Can you work these out from the model? Positions are in its coordinate system, mm. Face numbers are marked on the shaded views. Give positions to 0.01 mm unless a question says otherwise; leave off trailing zeros. Write each loop counter-clockwise with the first axis right and the second up, starting at its lowest first coordinate (ties: lowest second). Pieces come first, ordered by that corner, then holes.
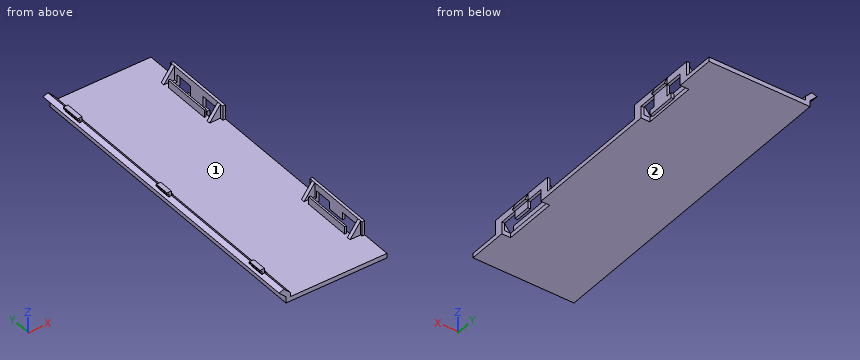
Autodesk Fusion 360 part; units mm, degrees
sketch "Sketch1" plane through (0, 0, 0) normal (0, 0, 1) x (1, 0, 0)
  line L0 (27, 90) -> (-27, 90)
  line L1 (-27, 90) -> (-27, -90)
  line L2 (-27, -90) -> (27, -90)
  line L3 (27, -90) -> (27, 90)
  dimension "d1" = 54
  dimension "d2" = 180
extrude "Extrude1" add sketch "Sketch1" along normal blind 2.5
sketch "Sketch2" plane through (0, 90, 0) normal (0, 1, 0) x (-1, 0, 0)
  line L0 (-27, 0) -> (27, 0)
  line L1 (27, 0) -> (27, 2.5)
  line L2 (27, 2.5) -> (-27, 2.5)
  line L3 (-27, 2.5) -> (-27, 0)
  line L4 (27, 0) -> (29.5, 0)
  line L5 (29.5, 0) -> (29.5, 2.5)
  line L6 (27, 2.5) -> (27, 4.8)
  line L7 (29.5, 0) -> (29.5, 3.5)
  line L8 (29.5, 3.5) -> (33.3891, 7.3891)
  line L9 (27, 4.8) -> (30.5355, 8.3355)
  line L10 (27, 4.8) -> (32.5, 4.8) construction
  line L11 (30.5355, 8.3355) -> (33.3891, 7.3891)
  dimension "d5" = 2.5
  dimension "d6" = 2.5
  dimension "d7" = 2.3
  dimension "d8" = 135
  dimension "d9" = 5.5
  dimension "d10" = 45
  dimension "d11" = 5
extrude "Extrude2" add sketch "Sketch2" against normal blind 180 contours L1 L4 L5 L6 L7 L8 L9 L11
sketch "Sketch3" plane through (0, 90, 0) normal (0, 1, 0) x (-1, 0, 0)
  line L0 (-27, 0) -> (29.5, 0)
  line L1 (29.5, 0) -> (29.5, 3.5)
  line L2 (29.5, 3.5) -> (33.3891, 7.3891)
  line L3 (33.3891, 7.3891) -> (30.5355, 8.3355)
  line L4 (30.5355, 8.3355) -> (27, 4.8)
  line L5 (27, 4.8) -> (27, 2.5)
  line L6 (27, 2.5) -> (-27, 2.5)
  line L7 (-27, 2.5) -> (-27, 0)
  line L8 (31.8891, 8.3429) -> (31.8891, 7.8866)
  line L9 (31.8891, 8.3429) -> (31.8891, 9.8429)
  line L10 (31.8891, 9.8429) -> (33.0391, 9.8429)
  line L11 (33.1891, 9.9929) -> (33.1891, 10.6929)
  line L12 (33.0391, 10.8429) -> (30.5355, 10.8429)
  line L13 (30.5355, 10.8429) -> (30.5355, 8.3355)
  arc A0 (33.1891, 10.6929) -> (33.0391, 10.8429) centre (33.0391, 10.6929) ccw
  arc A1 (33.0391, 9.8429) -> (33.1891, 9.9929) centre (33.0391, 9.9929) ccw
  line L14 (30.5355, 10.8429) -> (27, 4.8)
  point P0 (33.1891, 9.8429)
  point P1 (33.1891, 10.8429)
  dimension "d15" = 1.5
  dimension "d16" = 1.3
  dimension "d17" = 1
  dimension "d19" = 0.15
  dimension "d24" = 1.5
extrude "Extrude3" add sketch "Sketch3" along normal blind -26 and the other way blind 15.2 contours L3 L8 L9 L10 L11 L12 L13 A0 A1
extrude "Extrude4" add sketch "Sketch3" along normal blind -20 and the other way blind 22 contours L4 L13 L14
extrude "Extrude5" add sketch "Sketch3" along normal blind -94 and the other way blind 86 contours L3 L8 L9 L10 L11 L12 L13 A0 A1
extrude "Extrude6" add sketch "Sketch3" along normal blind -157 and the other way blind 165 contours L3 L8 L9 L10 L11 L12 L13 A0 A1
extrude "Extrude7" add sketch "Sketch3" along normal blind -162 and the other way blind 160 contours L4 L13 L14
extrude "Extrude8" add sketch "Sketch3" along normal blind -89 and the other way blind 91 contours L4 L13 L14
sketch "Sketch4" plane through (27, 0, 0) normal (1, 0, 0) x (0, 0, -1)
  line L0 (0, -90) -> (0, 90)
  line L1 (0, 90) -> (-2.5, 90)
  line L2 (-2.5, 90) -> (-2.5, -90)
  line L3 (-2.5, -90) -> (0, -90)
  line L4 (-2.5, -90) -> (-2.5, -73)
  line L5 (-2.5, -73) -> (-10.5, -73)
  line L6 (-10.5, -73) -> (-10.5, -33.2)
  line L7 (-2.5, -73) -> (-2.5, -68)
  line L8 (-2.5, -68) -> (-6.7, -68)
  line L9 (-10.5, -33.2) -> (-2.5, -33.2)
  line L10 (-6.7, -68) -> (-6.7, -58)
  line L11 (-6.7, -58) -> (-0.2, -58)
  line L12 (-0.2, -58) -> (-0.2, -61.1)
  line L13 (-0.2, -61.1) -> (2.7, -61.1)
  line L14 (2.7, -61.1) -> (2.7, -45.1)
  line L15 (-0.2, -48.2) -> (-0.2, -45.1)
  line L16 (-0.2, -45.1) -> (2.7, -45.1)
  line L17 (-6.7, -48.2) -> (-0.2, -48.2)
  line L18 (-6.7, -38.2) -> (-6.7, -48.2)
  line L19 (-2.5, -33.2) -> (-2.5, -38.2)
  line L20 (-2.5, -38.2) -> (-6.7, -38.2)
  line L21 (2.7, -61.1) -> (2.7, -69)
  line L22 (-2.5, -68) -> (2.7, -68)
  line L23 (-2.5, -38.2) -> (3, -38.2)
  line L24 (2.7, -45.1) -> (2.7, -38.2)
  line L25 (-1.75, 0) -> (-22.5, 0)
  line L26 (-0.2, 48.2) -> (-0.2, 45.1)
  line L27 (-0.2, 61.1) -> (2.7, 61.1)
  line L28 (-10.5, 73) -> (-10.5, 33.2)
  line L29 (-0.2, 58) -> (-0.2, 61.1)
  line L30 (-2.5, 38.2) -> (3, 38.2)
  line L31 (2.7, 61.1) -> (2.7, 69)
  line L32 (-6.7, 68) -> (-6.7, 58)
  line L33 (2.7, 61.1) -> (2.7, 45.1)
  line L34 (-6.7, 38.2) -> (-6.7, 48.2)
  line L35 (2.7, 45.1) -> (2.7, 38.2)
  line L36 (-10.5, 33.2) -> (-2.5, 33.2)
  line L37 (-2.5, 68) -> (-6.7, 68)
  line L38 (-2.5, 73) -> (-2.5, 68)
  line L39 (-6.7, 48.2) -> (-0.2, 48.2)
  line L40 (-0.2, 45.1) -> (2.7, 45.1)
  line L41 (-2.5, 68) -> (2.7, 68)
  line L42 (-2.5, 38.2) -> (-6.7, 38.2)
  line L43 (-2.5, 33.2) -> (-2.5, 38.2)
  line L44 (-2.5, 73) -> (-10.5, 73)
  line L45 (-6.7, 58) -> (-0.2, 58)
  dimension "d45" = 17
  dimension "d46" = 8
  dimension "d47" = 39.8
  dimension "d48" = 4.2
  dimension "d50" = 6.5
  dimension "d51" = 3.1
  dimension "d52" = 2.9
extrude "Extrude9" cut sketch "Sketch4" against normal blind 4.9 contours L0 L2 L11 L12 L13 L22 | L0 L13 L21 L22 | L0 L2 L11 L12 L13 L15 L16 L17 | L0 L13 L14 L16 | L2 L8 L10 L11 | L0 L2 L15 L16 L17 L23 | L0 L16 L23 L24 | L2 L17 L18 L20 | L0 L2 L26 L30 L39 L40 | L0 L30 L35 L40 | L0 L2 L26 L27 L29 L39 L40 L45 | L0 L27 L33 L40 | L2 L34 L39 L42 | L0 L2 L27 L29 L41 L45 | L0 L27 L31 L41 | L2 L32 L37 L45
extrude "Extrude10" add sketch "Sketch4" against normal blind 1.5 contours L0 L2 L11 L12 L13 L15 L16 L17 | L0 L13 L14 L16 | L2 L5 L6 L7 L8 L9 L10 L11 L17 L18 L19 L20
sketch "Sketch5" plane through (0, -73, 0) normal (0, -1, 0) x (1, 0, 0)
  line L0 (27, 2.5) -> (27, 10.5)
  line L1 (27, 10.5) -> (25.5, 10.5)
  line L2 (25.5, 10.5) -> (25.5, 2.5)
  line L3 (25.5, 2.5) -> (27, 2.5)
  line L4 (27, 10.5) -> (27, 6.7)
  line L5 (27, 6.7) -> (28.5, 6.7)
  line L6 (28.5, 6.7) -> (27, 10.5)
extrude "Extrude11" add sketch "Sketch5" along normal blind -24.8 and the other way blind 15 contours L0 L4 L5 L6
sketch "Sketch6" plane through (0, -73, 0) normal (0, -1, 0) x (1, 0, 0)
  line L0 (27, 2.5) -> (27, 10.5)
  line L1 (27, 10.5) -> (25.5, 10.5)
  line L2 (25.5, 10.5) -> (25.5, 2.5)
  line L3 (25.5, 2.5) -> (27, 2.5)
  line L4 (27, 2.5) -> (14.9732, 2.5)
  line L5 (25.5, 10.5) -> (19.5, 2.5)
  point P0 (25.5, 2.5)
  dimension "d62" = 6
extrude "Extrude12" add sketch "Sketch6" along normal blind -3 and the other way blind 1 contours L2 L4 L5
extrude "Extrude13" add sketch "Sketch6" along normal blind -38 and the other way blind 36 contours L2 L4 L5
sketch "Sketch7" plane through (0, 0, 2.5) normal (0, 0, 1) x (1, 0, 0)
  line L0 (19.5, -35) -> (25.5, -35)
  line L1 (25.5, -35) -> (25.5, -33.2)
  line L2 (25.5, -33.2) -> (27, -33.2)
  line L3 (27, -33.2) -> (27, 38.2)
  line L4 (27, 90) -> (-27, 90)
  line L5 (-27, 90) -> (-27, -90)
  line L6 (-27, -90) -> (27, -90)
  line L7 (27, -90) -> (27, -73)
  line L8 (27, -73) -> (25.5, -73)
  line L9 (25.5, -73) -> (25.5, -72)
  line L10 (25.5, -72) -> (19.5, -72)
  line L11 (19.5, -72) -> (19.5, -70)
  line L12 (19.5, -70) -> (25.5, -70)
  line L13 (25.5, -70) -> (25.5, -68)
  line L14 (25.5, -68) -> (22.1, -68)
  line L15 (22.1, 38.2) -> (22.1, 68)
  line L16 (22.1, -38.2) -> (25.5, -38.2)
  line L17 (25.5, -38.2) -> (25.5, -37)
  line L18 (25.5, -37) -> (19.5, -37)
  line L19 (19.5, -37) -> (19.5, -35)
  line L20 (20, -37) -> (20, -39.8)
  line L21 (20, -70) -> (20, -67.2)
  line L22 (20, -39.8) -> (21, -39.8)
  line L23 (21, -39.8) -> (21, -67.4697)
  line L24 (20, -67.2) -> (21, -67.2)
  line L25 (20, -67.2) -> (20, -39.8)
  line L26 (27, 38.2) -> (22.1, 38.2)
  line L27 (22.1, 68) -> (27, 68)
  line L28 (27, 68) -> (27, 90)
  line L29 (22.1, -68) -> (22.1, -38.2)
  dimension "d71" = 2.8
  dimension "d72" = 2.8
extrude "Extrude14" add sketch "Sketch7" along normal blind 4.2 contours L22 L23 L24 L25
mirror "Mirror1" about plane through (0, 0, 0) normal (0, 1, 0) of "Extrude1", "Extrude9", "Extrude10", "Extrude11", "Extrude12", "Extrude13", "Extrude14"
(1) Will these pins go through, and if not, where does the flat tip stop? P1, Ø1.5, axis at x = -4, z = -1, coming from the -Y side; P2, Ø1.2, axis at x = 26.5, z = -1, coming from the -Y side; P3, Ø5, axis at x = 24, z = 5.5, coming from the +Y side; P4, Ø4, axis at x = -28, z = 9, coming from the -Y side.
Returned:
P1: passes through
P2: stops at y = 45.1
P3: stops at y = 73
P4: stops at y = -72
(2) Imagine slicing it at B-B, the plane x = 7. Write out the boundary of the cut face in (y, z).
Returned:
outline: (-90, 0) - (90, 0) - (90, 2.5) - (-90, 2.5) - close
(3) If we mould it in two halves opening along X, with no side actions, what happens to the marked faces 1 and 2? For each: +X half, -X half, draft (parallel to the pull), parting line (faces both ways), or undercut.
Returned:
face 1: undercut
face 2: draft
(4) If I drill on L1, parallel to Y at x = 26.5, z = 4.5; L2, parallel to Z at x = 10, y = -26.5; L3, parallel to X at y = -66.5, z = 0.5, over which ranges is the centre line in solid material (lowest first)?
Returned:
L1: y = -73 to -68, -58 to -48.2, -38.2 to -33.2, 33.2 to 38.2, 48.2 to 58, 68 to 73
L2: z = 0 to 2.5
L3: x = -29.5 to 22.1
(5) Imagine slicing it at A-A, the plane y = -60.5. Write out the boundary of the cut face in (x, z).
Returned:
outline: (-33.39, 7.39) - (-29.5, 3.5) - (-29.5, 0) - (22.1, 0) - (22.1, 2.5) - (21, 2.5) - (21, 6.7) - (20, 6.7) - (20, 2.5) - (-27, 2.5) - (-27, 4.8) - (-30.54, 8.34) - close; (25.5, 6.7) - (27, 6.7) - (27, 10.5) - (25.5, 10.5) - close
